Design review of the part built by this model. Coordinates are the model's own, in mm. Face numbers are marked on the shaded views. Give positions to 0.01 mm unless a question says otherwise; leave off trailing zeros. Loops run counter-clockwise (first coordinate to the right, second up) from the corner with the lowest first, then second, coordinate; pieces in that order, holes last. Notation, with made-up numbers: (-25, 49) - (18, 49) arc R14 cw to (18, 71) - close; hole circle Ø5 at (64.25, 3). An arc over 180 degrees is marked (long way). Write each question's results on one line, items separated by ' | '.
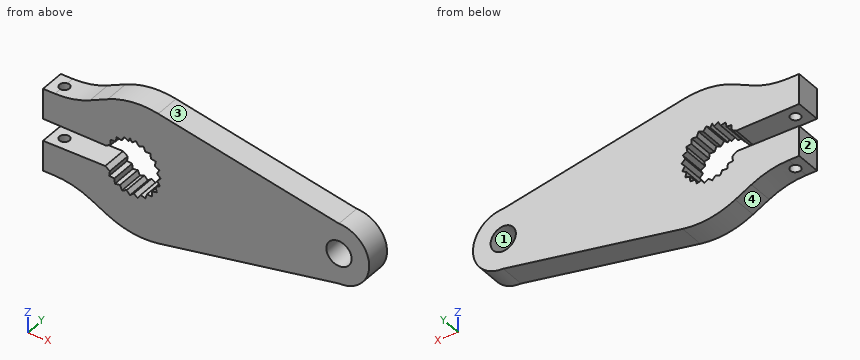
from build123d import *

# Parameters (mm, degrees)
BOSS_EXTRUDE1_DEPTH     = 6.35
CUT_EXTRUDE1_REACH      = 46.798
SKETCH2_R               = 3.175
CUT_EXTRUDE2_DEPTH      = 45.797927572
CUT_EXTRUDE2_DEPTH_BACK = 45.797927572
SKETCH3_R               = 1.27


with BuildPart() as part:
    # Sketch1 → Boss-Extrude1 (new body)
    with BuildSketch(Plane(origin=(0, 0, 0), x_dir=(1, 0, 0), z_dir=(0, 1, 0))):
        with BuildLine():
            Line((-25.172750094, -2.854782141), (-23.979365131, -3.554335257))
            Line((-23.979365131, -3.554335257), (-24.045420885, -4.814754144))
            Line((-24.045420885, -4.814754144), (-22.785001999, -4.880809899))
            Line((-22.785001999, -4.880809899), (-22.501080336, -6.110609729))
            Line((-22.501080336, -6.110609729), (-21.271280506, -5.826688067))
            Line((-21.271280506, -5.826688067), (-20.659378714, -6.930588121))
            Line((-20.659378714, -6.930588121), (-19.555478659, -6.318686329))
            Line((-19.555478659, -6.318686329), (-19.145844879, -7.284635532))
            Line((-19.145844879, -7.284635532), (-18.663004813, -6.38109418))
            Line((-18.663004813, -6.38109418), (-17.655008108, -7.140674179))
            Line((-17.655008108, -7.140674179), (-16.895428108, -6.132677474))
            Line((-16.895428108, -6.132677474), (-15.717110864, -6.584991086))
            Line((-15.717110864, -6.584991086), (-15.264797252, -5.406673842))
            Line((-15.264797252, -5.406673842), (-14.00745149, -5.516677342))
            Line((-14.00745149, -5.516677342), (-13.89744799, -4.259331581))
            Line((-13.89744799, -4.259331581), (-12.658488598, -4.018502271))
            Line((-12.658488598, -4.018502271), (-12.899317907, -2.779542878))
            Line((-12.899317907, -2.779542878), (-11.774735254, -2.206539397))
            Line((-11.774735254, -2.206539397), (-12.347738736, -1.081956744))
            Line((-12.347738736, -1.081956744), (-11.424661673, -0.221173456))
            Line((-11.424661673, -0.221173456), (-12.28544496, 0.701903607))
            Line((-12.28544496, 0.701903607), (-11.635390366, 1.783776131))
            Line((-11.635390366, 1.783776131), (-12.717262889, 2.433830725))
            Line((-12.717262889, 2.433830725), (-12.390594789, 3.652972671))
            Line((-12.390594789, 3.652972671), (-13.609736736, 3.979640771))
            Line((-13.609736736, 3.979640771), (-13.631764267, 5.241597158))
            Line((-13.631764267, 5.241597158), (-14.893720653, 5.219569627))
            Line((-14.893720653, 5.219569627), (-15.262737196, 6.426568353))
            Line((-15.262737196, 6.426568353), (-16.469735922, 6.05755181))
            Line((-16.469735922, 6.05755181), (-17.157151327, 7.116078708))
            Line((-17.157151327, 7.116078708), (-18.215678225, 6.428663303))
            Line((-18.215678225, 6.428663303), (-19.168233878, 7.256707299))
            Line((-19.168233878, 7.256707299), (-19.996277875, 6.304151646))
            Line((-19.996277875, 6.304151646), (-21.140172995, 6.837558701))
            Line((-21.140172995, 6.837558701), (-21.67358005, 5.69366358))
            Line((-21.67358005, 5.69366358), (-22.920189524, 5.891107124))
            Line((-22.920189524, 5.891107124), (-23.117633068, 4.64449765))
            Line((-23.117633068, 4.64449765), (-24.370373821, 4.490680427))
            Line((-24.370373821, 4.490680427), (-24.216556598, 3.237939674))
            Line((-24.216556598, 3.237939674), (-25.378370526, 2.412676209))
            Line((-25.378370526, 2.412676209), (-41.02702196, 2.557572596))
            Line((-41.02702196, 2.557572596), (-41.02702196, 10.177572596))
            Line((-41.02702196, 10.177572596), (-38.355583111, 10.177572596))
            ThreePointArc((-38.355583111, 10.177572596), (-33.547545085, 10.754594848), (-29.012572504, 12.452890476))
            Line((-29.012572504, 12.452890476), (-24.949455261, 14.556654192))
            ThreePointArc((-24.949455261, 14.556654192), (-18.492857296, 16.625923003), (-11.714907277, 16.455851756))
            Line((-11.714907277, 16.455851756), (33.40702196, 7.651462795))
            ThreePointArc((33.40702196, 7.651462795), (41.02702196, 0.031462795), (33.40702196, -7.588537205))
            Line((33.40702196, -7.588537205), (-12.038677684, -16.4558708))
            ThreePointArc((-12.038677684, -16.4558708), (-18.523682802, -16.66577615), (-24.744249109, -14.820808279))
            Line((-24.744249109, -14.820808279), (-29.229404705, -12.661591197))
            ThreePointArc((-29.229404705, -12.661591197), (-33.523201838, -11.159597642), (-38.043536354, -10.650427404))
            Line((-38.043536354, -10.650427404), (-41.02702196, -10.650427404))
            Line((-41.02702196, -10.650427404), (-41.02702196, -3.030427404))
            Line((-41.02702196, -3.030427404), (-25.172750094, -2.854782141))
        make_face()
    extrude(amount=BOSS_EXTRUDE1_DEPTH)

    # Sketch2 → Cut-Extrude1 (cut, up to next)
    with BuildSketch(Plane(origin=(0, 6.35, 0), x_dir=(1, 0, 0), z_dir=(0, 1, 0)), mode=Mode.PRIVATE) as cut_extrude1_sk1:
        with Locations(Location((33.40702196, 0.031462795, 0), (0, 0, 270))):
            Circle(SKETCH2_R)
    cut_extrude1_tool1 = extrude(cut_extrude1_sk1.sketch, amount=-CUT_EXTRUDE1_REACH, mode=Mode.PRIVATE) & part.part
    add(cut_extrude1_tool1.solids().sort_by_distance((33.407022, 6.35, -0.031463))[0], mode=Mode.SUBTRACT)

    # Sketch3 → Cut-Extrude2 (cut, two sides: drawn at the far end of the back side and taken through both)
    with BuildSketch(Plane.XY.offset(-CUT_EXTRUDE2_DEPTH_BACK)):
        with Locations((-37.85202196, 3.175)):
            Circle(SKETCH3_R)
    extrude(amount=CUT_EXTRUDE2_DEPTH + CUT_EXTRUDE2_DEPTH_BACK, mode=Mode.SUBTRACT)


solid = part.part
(1) Take a section at C-C on x = 31. Give the boundary of the cut face in (y, z).
Answers below:
outline: (0, -8.12) - (6.35, -8.12) - (6.35, -2.1) - (0, -2.1) - close; (0, 2.04) - (6.35, 2.04) - (6.35, 8.06) - (0, 8.06) - close
(2) Insertion check: P1, Ø4, axis at x = 13.5, z = -10, coming from the -Y side; P2, Ø1.5, axis at x = -39, y = 2, coming from the +Z side; P3, Ø2, axis at x = 7, y = 3.5, coming from the +Z side; P4, Ø5.5, axis at x = 33.41, z = -0.03, coming from the +Y side. Each pin has a flat end and moves straight along its axis. Give the tip position at first contact, or say it passes through.
Answers below:
P1: y = 0 | P2: z = 10.65 | P3: z = 12.94 | P4: through
(3) Take a section at D-D on x = -5. Give the boundary of the cut face in (y, z).
Answers below:
outline: (0, -15.15) - (6.35, -15.15) - (6.35, 15.08) - (0, 15.08) - close
(4) Draft analysis for pull direction Z (two halves, no side actions). For the marked faces 1, 2, 3 and 4, state which applies: pulls with the +Z half, pulls with the -Z half, needs draft (parallel to the pull), parting line crosses it, or undercut.
Answers below:
face 1: undercut | face 2: needs draft | face 3: pulls with the +Z half | face 4: pulls with the -Z half
(5) Take a section at A-A on x = -33.5. Give the boundary of the cut face in (y, z).
Answers below:
outline: (0, -10.77) - (6.35, -10.77) - (6.35, -2.49) - (0, -2.49) - close; (0, 2.95) - (6.35, 2.95) - (6.35, 11.16) - (0, 11.16) - close
(6) Take a section at B-B on z = 9.5. Give the boundary of the cut face in (x, y) (3 decimals), plus the area to 3 significant figures.
Answers below:
outline: (-41.027, 0) - (23.611, 0) - (23.611, 6.35) - (-41.027, 6.35) - close; hole circle Ø2.54 at (-37.852, 3.175) | area: 405 mm2
(7) Wall thickness on line 1 along X through (y, z) = (2.25, 5); line 2 along Z through (x, y) = (32, 3); line 3 along Z through (x, y) = (-28, 4.75): over which ranges is each line inside the solid? List them lowest first. Write a range as from..to.
Answers below:
line 1: -41.03..-38.72, -36.98..-22.76, -13.96..39.13 | line 2: -7.93..-2.88, 2.81..7.86 | line 3: -12.98..-2.44, 2.89..13.25
